Geometry: final body of the model. Coordinates: model frame, mm. Face numbers are marked on the shaded views. A direction names the side the tool comes from. Round coordinates to 2 decimals unless told otherwise and drop trailing zeros. Loops run counter-clockwise (first coordinate to the right, second up) from the corner with the lowest first, then second, coordinate; pieces in that order, holes last. Notation, with made-up numbers: (84.25, 55) - (130.25, 55) arc R22 ccw to (130.25, 91) - close; hole circle Ø5 at (42, 17.5). An arc over 180 degrees is marked (long way). Return JSON: item names as keys, results as strings. Group by question number.
1. Section D-D on y = 10.5. Return loops of the section in (x, z).
2. First-contact query: pin 1 Ø4 at (x, y) = (-12, 10) entering from -Z; pin 2 Ø2.5 at (x, y) = (11.5, 7) entering from -Z; pin 3 Ø9.5 at (y, z) = (8, -1.5) entering from -X; pin 4 Ø3 at (x, y) = (-9, 8) entering from -Z. Flat tips, straight axial feed; report the tip coordinate or a pass-through.
3. Section A-A on x = 8.89. Return loops of the section in (y, z).
4. Set-up query: the marked faces 1, 2 and 3. Return all of +Z, -Z, +X, -X, +Y, -Y with unobstructed straight access to the full face (end or side cutting, diameter ignored); none if empty.
5. Section B-B on z = 5.08. Return loops of the section in (x, y), and give its area (3 significant figures).
6. Section C-C on y = -0.5. Return loops of the section in (x, z).
7. Material intervals for probe 1 along Y at (x, z) = (-9.75, 6.5); probe 2 along Z at (x, y) = (-9.25, 1); probe 3 along X at (y, z) = (4.5, -1), sorted ascending.
Autodesk Inventor part; units mm, degrees
ref_plane "YZ Plane" through (0, 0, 0) normal (1, 0, 0) x (0, 1, 0)
ref_plane "XZ Plane" through (0, 0, 0) normal (0, 1, 0) x (-1, 0, 0)
ref_plane "XY Plane" through (0, 0, 0) normal (0, 0, 1) x (1, 0, 0)
sketch "Sketch1" plane through (0, 0, 0) normal (0, 1, 0) x (-1, 0, 0)
  line L0 (13.75, 16.25) -> (-13.75, 16.25)
  line L1 (-13.75, 16.25) -> (-13.75, -16.25)
  line L2 (-13.75, -16.25) -> (13.75, -16.25)
  line L3 (13.75, -16.25) -> (13.75, 16.25)
  line L4 (-13.75, 0.7762) -> (-9.8958, 0.7762)
  line L5 (-9.8958, 0.7762) -> (-9.8958, -16.25)
  line L6 (13.75, 3.9572) -> (7.9724, 3.9572)
  line L7 (7.9724, 3.9572) -> (7.9724, -16.25)
  point P0 (0, 0)
  dimension "d0" = 27.5
  dimension "d1" = 13.75
  dimension "d2" = 32.5
  dimension "d3" = 16.25
extrude "Extrusion1" add sketch "Sketch1" along normal blind 20.8 contours L3 L6 L7 L2 L5 L4 L1 L0
sketch "Sketch2" plane through (0, 0, 0) normal (0, -1, 0) x (1, 0, 0)
  circle A0 centre (-8.89, 7.62) radius 0.8
  circle A1 centre (8.89, 5.08) radius 0.8
  circle A2 centre (-5.08, -7.62) radius 0.32
  circle A3 centre (5.08, -7.62) radius 0.32
  point P0 (0, 0)
  dimension "d6" = 0.64
  dimension "d7" = 0.64
  dimension "d8" = 3.81
  dimension "d9" = 13.97
  dimension "d10" = 17.78
  dimension "d11" = 2.54
  dimension "d12" = 15.24
  dimension "d13" = 0
  dimension "d14" = 5.08
  dimension "d15" = 7.62
  dimension "d16" = 1.6
  dimension "d17" = 1.6
extrude "Extrusion2" add sketch "Sketch2" along normal blind 3.6
fillet "Fillet1" radius 0.5 15 edges at (-7.9724, 10.4, 3.9572) (-7.9724, 10.4, -16.25) (-13.75, 10.4, 3.9572) (-13.75, 10.4, 16.25) (9.8958, 10.4, -16.25) (13.75, 10.4, 0.7762) (9.8958, 10.4, 0.7762) (0, 20.8, 16.25) (-13.75, 20.8, 10.1036) (-10.8612, 20.8, 3.9572) (-7.9724, 20.8, -6.1464) (0.9617, 20.8, -16.25) (9.8958, 20.8, -7.7369) (11.8229, 20.8, 0.7762) (13.75, 20.8, 8.5131)
properties part number "JTN1AS-PA-F-DC5V_Relay"
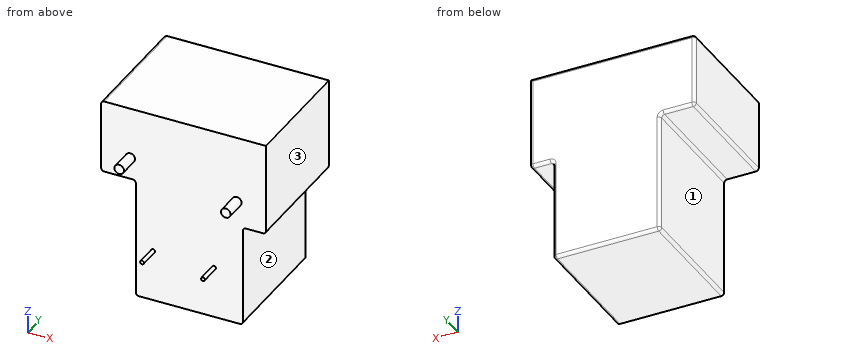
Taken from the geometry:
{
 "1": {"outline": "(-13.75, 4.46) arc R0.5 ccw to (-13.25, 3.96) - (-8.47, 3.96) arc R0.5 cw to (-7.97, 3.46) - (-7.97, -15.75) arc R0.5 ccw to (-7.47, -16.25) - (9.4, -16.25) arc R0.5 ccw to (9.9, -15.75) - (9.9, 0.28) arc R0.5 cw to (10.4, 0.78) - (13.25, 0.78) arc R0.5 ccw to (13.75, 1.28) - (13.75, 16.25) - (-13.25, 16.25) arc R0.5 ccw to (-13.75, 15.75) - close"},
 "2": {"pin 1": "z = 3.96", "pin 2": "z = 0.75", "pin 3": "x = -7.97", "pin 4": "z = -16.25"},
 "3": {"outline": "(-3.6, 4.28) - (0, 4.28) - (0, -16.25) - (20.3, -16.25) arc R0.5 ccw to (20.8, -15.75) - (20.8, 15.75) arc R0.5 ccw to (20.3, 16.25) - (0, 16.25) - (0, 5.88) - (-3.6, 5.88) - close"},
 "4": {"face 1": "-Z, -X, +Y, -Y", "face 2": "-Z, +X, +Y, -Y", "face 3": "+Z, -Z, +X, +Y, -Y"},
 "5": {"outline": "(-13.75, 0) - (8.09, 0) - (8.09, -3.6) - (9.69, -3.6) - (9.69, 0) - (13.75, 0) - (13.75, 20.3) arc R0.5 ccw to (13.25, 20.8) - (-13.25, 20.8) arc R0.5 ccw to (-13.75, 20.3) - close", "area": "578 mm2"},
 "6": {"outline": "circle Ø1.6 at (-8.89, 7.62); circle Ø0.64 at (-5.08, -7.62); circle Ø0.64 at (5.08, -7.62); circle Ø1.6 at (8.89, 5.08)"},
 "7": {"probe 1": "0 to 20.8", "probe 2": "3.96 to 16.25", "probe 3": "-7.97 to 9.9"}
}
